Part model, mm, in its own coordinate system. Coordinates: 2 decimals unless noted, no trailing zeros. Loops run counter-clockwise (first coordinate to the right, second up) from the corner with the lowest first, then second, coordinate; pieces in that order, holes last. Notation, with made-up numbers: (89.5, 79.5) -> (147.5, 79.5) arc R19 ccw to (147.5, 106.5) -> close; hole circle Ø11 at (-33, 6.5). An arc over 180 degrees is marked (long way). One line per item, written item: value. Start each with the question number.
from build123d import *

# Parameters (mm, degrees)
F0_W        = 33.9705549621
F0_H        = 87.9016891122
F1_DEPTH    = 17.9832
F2_T1_DEPTH = 127.9393629633
F3_T1_DEPTH = 181.1359395425


# Not quite as in the source:
# - a fillet or chamfer that OpenCascade refuses, or shapes differently, is made with other operations: its cross-section is extruded or revolved along the edge and cut away or added


with BuildPart() as f1:
    # F0 (on Top) → F1 (new body)
    with BuildSketch(Plane.XY):
        Rectangle(F0_W, F0_H)
    extrude(amount=-F1_DEPTH)

    # F2: chamfer of 12.9794 x 18.1964476933 on 2 edges, made by hand

    # F2_s2 → F2_t1 (cut)
    with BuildSketch(Plane.YZ.offset(-63.9696814817)):
        Polygon((-43.9508445561, 0.2132476933), (-30.9714445561, -17.9832), (-43.9508445561, -17.9832), align=None)
        Polygon((43.9508445561, 0.2132476933), (30.9714445561, -17.9832), (43.9508445561, -17.9832), align=None)
    extrude(amount=F2_T1_DEPTH, mode=Mode.SUBTRACT)

    # F3: chamfer of 4.826 x 18.0108771973 on 1 edges, made by hand

    # F3_s2 → F3_t1 (cut)
    with BuildSketch(Plane.XZ.offset(-90.5679697713)):
        Polygon((12.1592774811, 0), (16.9852774811, -18.0108771973), (16.9852774811, 0), align=None)
    extrude(amount=F3_T1_DEPTH, mode=Mode.SUBTRACT)


solid = f1.part
1) Slice it at B-B (x = -1). Give the cut face in (y, z).
2) Slice it at A-A (y = -2). Give the cut face in (x, z).
3) Pin check, flat tips, straight feed: pin 1 Ø10 at (y, z) = (3, -4) entering from +X; pin 2 Ø4 at (x, z) = (13.5, -7) entering from +Y; pin 3 Ø5 at (x, z) = (11.5, -10.5) entering from +Y; pin 4 Ø6 at (x, z) = (12.5, -2) entering from +Y. Stop position of each tip, or through.
4) Probe line 1 (X direction, y = -14, z = -7.75); line 2 (Y direction, x = 5, z = -15.75); line 3 (Y direction, x = 13.5, z = -11.5). List the from-to ranges inside material, lowest first. Write a range as from..to.
Check sheet entries:
1. outline: (-43.8, 0) -> (-30.97, -17.98) -> (30.97, -17.98) -> (43.8, 0) -> close
2. outline: (-16.99, -17.98) -> (16.98, -17.98) -> (12.16, 0) -> (-16.99, 0) -> close
3. pin 1: stops at x = 14.57
3. pin 2: stops at y = 40.23
3. pin 3: stops at y = 38.09
3. pin 4: stops at y = 43.8
4. line 1: x = -16.99..14.24
4. line 2: y = -32.56..32.56
4. line 3: y = -35.6..35.6
